Could you check a few things on this drawing? It's one solid part, dimensions in mm from its lowest x, y, z. A direction names the side the tool comes from. Give positions to 0.01 mm unless a question says otherwise; leave off trailing zeros. Order: outer loops, then holes, each group sorted by start corner. A loop starts at its lowest first (then second) coordinate and runs counter-clockwise, first axis right, second up. Notation, with made-up numbers: (58, 18) -> (68, 18) arc R16 ccw to (68, 40) -> close; hole circle Ø1 at (30, 51). An arc over 180 degrees is marked (long way). Use one line per item in the form item = value. Start each with the question number.
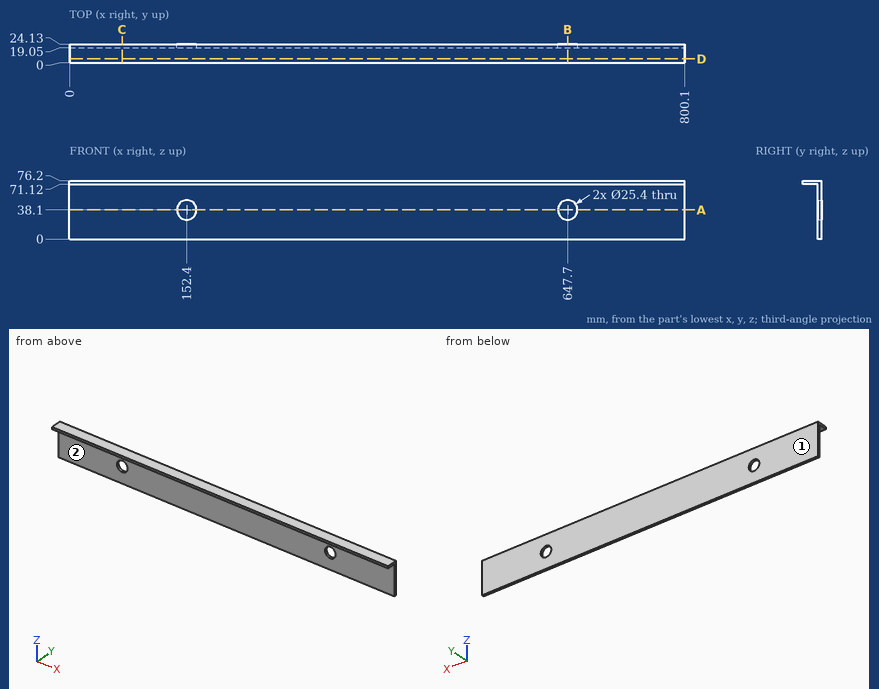
(1) Imagine slicing it at B-B (x = 647.7). Write out the boundary of the cut face in (y, z), plus the area to 3 significant figures.
(2) Imagine slicing it at C-C (x = 68.5). Write out the boundary of the cut face in (y, z), plus the area to 3 significant figures.
(3) Imagine slicing it at D-D (y = 4.75). Write out the boundary of the cut face in (x, z), plus the area to 3 significant figures.
(4) Which directions (+Z, -Z, +X, -X, +Y, -Y) give clear straight access to the entire face, cutting with the end or side of a thin tool? Please do the marked faces 1 and 2.
(5) Please list where these lines run through material, in increasing order: probe 1 along Z at (x, y) = (152.4, 21.85); probe 2 along Z at (x, y) = (313.5, 3.75); probe 3 along Y at (x, z) = (595, 65.5).
(6) Imagine slicing it at A-A (z = 38.1). Write out the boundary of the cut face in (x, y), plus the area to 3 significant figures.
(7) I'm going to push flat-ended pins straight in: pin 1 Ø1 at (x, z) = (588, 10) entering from -Y; pin 2 Ø5 at (x, y) = (711, 14) entering from -Z. Where does each tip first touch, or does it pass through?
Calculated:
q1.outline = (0, 71.12) -> (19.05, 71.12) -> (19.05, 50.8) -> (24.13, 50.8) -> (24.13, 76.2) -> (0, 76.2) -> close; (19.05, 0) -> (24.13, 0) -> (24.13, 25.4) -> (19.05, 25.4) -> close
q1.area = 355 mm2
q2.outline = (0, 71.12) -> (19.05, 71.12) -> (19.05, 0) -> (24.13, 0) -> (24.13, 76.2) -> (0, 76.2) -> close
q2.area = 484 mm2
q3.outline = (0, 71.12) -> (800.1, 71.12) -> (800.1, 76.2) -> (0, 76.2) -> close
q3.area = 4,060 mm2
q4.face_1 = +Z, -Z, +X, -X, +Y
q4.face_2 = -Z, +X, -X, -Y
q5.probe_1 = 0 to 25.4, 50.8 to 76.2
q5.probe_2 = 71.12 to 76.2
q5.probe_3 = 19.05 to 24.13
q6.outline = (0, 19.05) -> (139.7, 19.05) -> (139.7, 24.13) -> (0, 24.13) -> close; (165.1, 19.05) -> (635, 19.05) -> (635, 24.13) -> (165.1, 24.13) -> close; (660.4, 19.05) -> (800.1, 19.05) -> (800.1, 24.13) -> (660.4, 24.13) -> close
q6.area = 3,810 mm2
q7.pin_1 = 19.05
q7.pin_2 = 71.12
